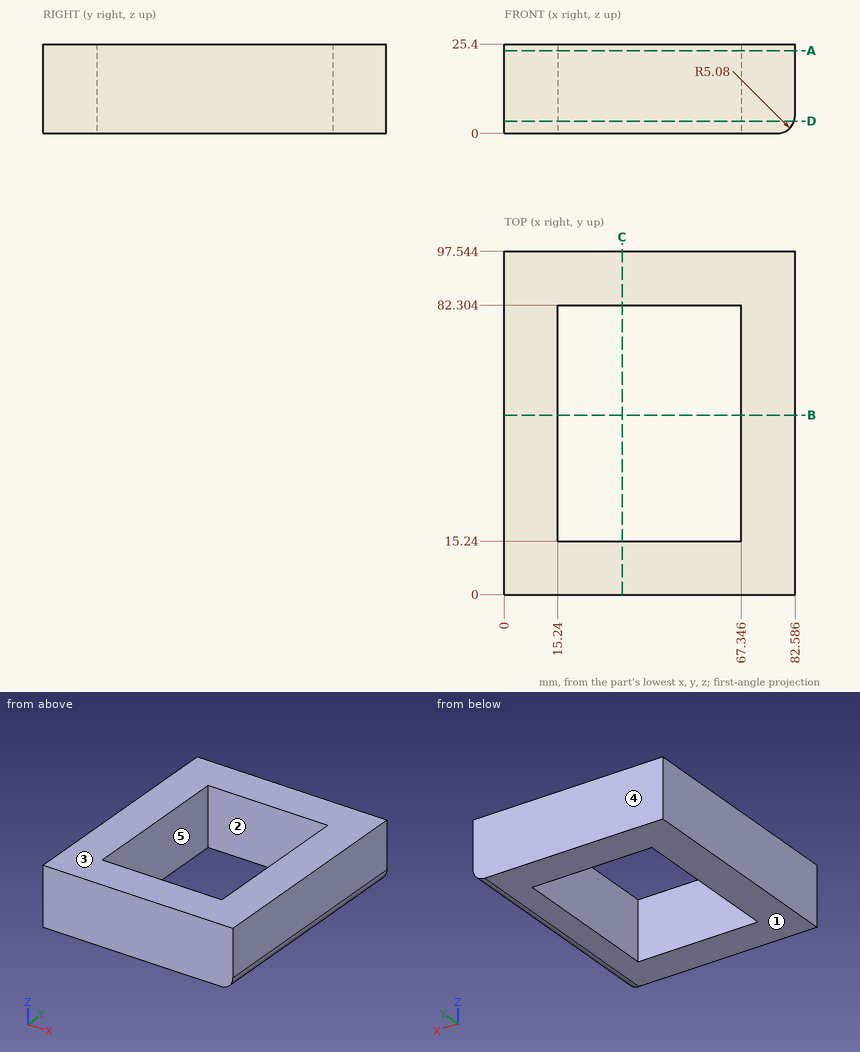
Print and shaded views of the part. All mm, measured from the part's lowest x, y and z. A direction names the side the tool comes from. Give positions to 0.01 mm unless a question says otherwise; leave off trailing zeros. Loops run counter-clockwise (first coordinate to the right, second up) from the corner with the lowest first, then second, coordinate; pieces in that order, holes last. Notation, with made-up numbers: (42.25, 8) -> (52.25, 8) arc R31 cw to (52.25, 40) -> close; hole circle Ø8 at (-31.5, -16.5). An arc over 180 degrees is marked (long way). One line per question, with ' | ' between items. Start each with the question number.
1) Probe L1, parallel to X at y = 35, z = 15.75 (1 decimal); L2, parallel to Y at x = 55.5, z = 15.5; L3, parallel to X at y = 77.5, z = 1.75 (1 decimal). List the from-to ranges inside material, lowest first.
2) Pin check, flat tip, straight feed: pin 1 (10 mm diameter, centred on x = 61, y = 49.5, fed in from +Z). Stop position of the tip, or through.
3) Cut at D-D (z = 3.5). Give the cut face in (x, y) (1 decimal).
4) Two-plate mould, pull along Z, no slides. Class the marked faces 1, 2 and 3: released by +Z, released by -Z, zero draft, split by the parting line, or undercut.
5) Cut at C-C (x = 33.5). Give the cut face in (y, z).
6) 3-axis set-ups, long thin cutter, end or side, ignore diameter. For the marked faces 4 and 5: which of +Z, -Z, +X, -X, +Y, -Y reach the whole face in a straight line?
7) Cut at B-B (y = 51). Give the cut face in (x, z) (1 decimal).
8) Cut at A-A (z = 23.5). Give the cut face in (x, y) (1 decimal), plus the area to 3 significant figures.
Return value:
1) L1: 0 to 15.2, 67.3 to 82.6 | L2: 0 to 15.24, 82.3 to 97.54 | L3: 0 to 15.2, 67.3 to 81.3
2) pin 1: through
3) outline: (0, 0) -> (82.3, 0) -> (82.3, 97.5) -> (0, 97.5) -> close; hole (15.2, 15.2) -> (67.3, 15.2) -> (67.3, 82.3) -> (15.2, 82.3) -> close
4) face 1: released by -Z | face 2: zero draft | face 3: released by +Z
5) outline: (0, 0) -> (15.24, 0) -> (15.24, 25.4) -> (0, 25.4) -> close; (82.3, 0) -> (97.54, 0) -> (97.54, 25.4) -> (82.3, 25.4) -> close
6) face 4: +Z, -Z, +X, -X, +Y | face 5: +Z, -Z
7) outline: (0, 0) -> (15.2, 0) -> (15.2, 25.4) -> (0, 25.4) -> close; (67.3, 0) -> (77.5, 0) arc R5.1 ccw to (82.6, 5.1) -> (82.6, 25.4) -> (67.3, 25.4) -> close
8) outline: (0, 0) -> (82.6, 0) -> (82.6, 97.5) -> (0, 97.5) -> close; hole (15.2, 15.2) -> (67.3, 15.2) -> (67.3, 82.3) -> (15.2, 82.3) -> close | area: 4,560 mm^2
